For this review, use the dimensioned drawing (mm, ordinates from the lowest corner) and the shaded views. A direction names the side the tool comes from. Round coordinates to 2 decimals unless told otherwise and drop trailing zeros. Order: outer loops, then holes, each group sorted by start corner. A loop starts at its lowest first (then second) coordinate and runs counter-clockwise, first axis right, second up. Notation, with made-up numbers: (-19, 43.25) - (27, 43.25) arc R36 cw to (27, 77.25) - close; hole circle Ø7 at (-17, 28). An arc over 180 degrees is marked (long way). Use CSV: the item, a comma, the result in double quotes. Start each with the question number.
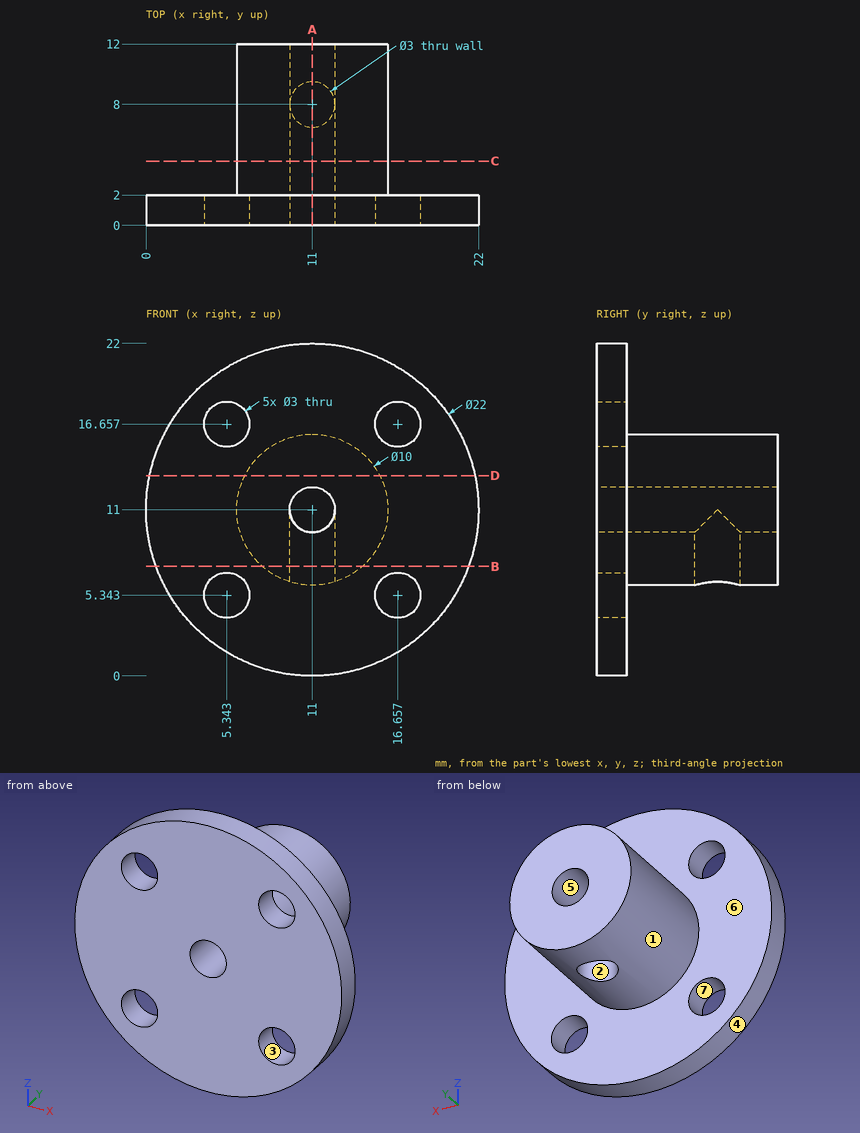
Q1. For L1, parallel to Z at x = 11, y = 3.5; L2, parallel to Y at x = 7.5, z = 14.75, list the stretches that pass through material, from the lowest coordinate up. Write a range as [from, to].
Q2. Take a section at D-D (z = 13.25). State the section outline as (x, y) points (1 decimal), plus the area to 3 significant figures.
Q3. Take a section at A-A (x = 11). State the section outline as (y, z) points.
Q4. Clearance check with flat-ended pins moving along their axes: pin 1 (3 mm diameter, centred on x = 14, y = 7.5, fed in from -Z); pin 2 (1.8 mm diameter, centred on x = 16.66, z = 5.34, fed in from +Y); pin 3 (2 mm diameter, centred on x = 2.5, z = 10.5, fed in from +Y); pin 4 (4 mm diameter, centred on x = 11, y = 8, fed in from -Z). State where each tip first meets the part, or that it passes through.
Q5. Take a section at B-B (z = 7.25). State the section outline as (x, y) points.
Q6. Tool access review of the marked faces 1, 2 and 3: name each direction out of +Z, -Z, +X, -X, +Y, -Y from which nothing blocks a thin tool from reaching the whole face with its end or side.
Q7. The part is to be moulded in two halves that separate along Z. For the marked faces 4, 5, 6 and 7, say which applies: +Z half, -Z half, draft (parallel to the pull), parting line (faces both ways), or undercut.
Q8. Take a section at C-C (y = 4.25). State the section outline as (x, z) points, plus the area to 3 significant figures.
Findings below:
1,L1,"z = [6, 9.5], [12.5, 16]"
1,L2,"y = [0, 2]"
2,outline,"(0.2, 0) - (21.8, 0) - (21.8, 2) - (15.5, 2) - (15.5, 12) - (6.5, 12) - (6.5, 2) - (0.2, 2) - close"
2,area,"132 mm^2"
3,outline,"(0, 0) - (2, 0) - (2, 6) - (6.5, 6) - (6.5, 9.5) - (0, 9.5) - close; (0, 12.5) - (12, 12.5) - (12, 16) - (2, 16) - (2, 22) - (0, 22) - close; (9.5, 6) - (12, 6) - (12, 9.5) - (9.5, 9.5) - close"
4,pin 1,"stops at z = 6.23"
4,pin 2,"passes through"
4,pin 3,"stops at y = 2"
4,pin 4,"stops at z = 6"
5,outline,"(0.66, 0) - (21.34, 0) - (21.34, 2) - (14.31, 2) - (14.31, 12) - (7.69, 12) - (7.69, 2) - (0.66, 2) - close; hole circle Ø3 at (11, 8)"
6,face 1,"+Y"
6,face 2,"-Z"
6,face 3,"+Y, -Y"
7,face 4,"parting line"
7,face 5,"undercut"
7,face 6,"draft"
7,face 7,"undercut"
8,outline,"circle Ø10 at (11, 11); hole circle Ø3 at (11, 11)"
8,area,"71.5 mm^2"
